from build123d import *

# Parameters (mm, degrees)
BOSS_EXTRU_1_DEPTH = 50
CONG_1_R           = 10


with BuildPart() as part:
    # Esquisse1 → Boss.-Extru.1 (new body)
    with BuildSketch(Plane(origin=(0, 0, 0), x_dir=(1, 0, 0), z_dir=(0, 1, 0))):
        with BuildLine():
            Line((0, 0), (-2, 0))
            ThreePointArc((-2, 0), (6.574510491, 25.388511074), (29, 40.058076335))
            Line((29, 40.058076335), (29, 50.058076335))
            Line((29, 50.058076335), (49, 50.058076335))
            Line((49, 50.058076335), (49, 40.058076335))
            ThreePointArc((49, 40.058076335), (71.425489509, 25.388511074), (80, 0))
            Line((80, 0), (78, 0))
            ThreePointArc((78, 0), (39, 39), (0, 0))
        make_face()
    extrude(amount=BOSS_EXTRU_1_DEPTH)

    # Congé1
    cong_1_edges = [part.edges().sort_by_distance(p)[0] for p in [
        (29, 25, -40.058076335),
        (49, 25, -40.058076335),
    ]]
    fillet(cong_1_edges, radius=CONG_1_R)


solid = part.part
Design review of the part built by this model. Coordinates are the model's own, in mm. A direction names the side the tool comes from. Coordinates: 2 decimals unless noted, no trailing zeros. Order: outer loops, then holes, each group sorted by start corner. A loop starts at its lowest first (then second) coordinate and runs counter-clockwise, first axis right, second up.
Item 1: For line 1 (X direction, y = 21, z = -29); line 2 (X direction, y = 7.5, z = -8); line 3 (X direction, y = 27, z = -47), list the stretches that pass through material, from the lowest coordinate up.
Item 2: Take a section at B-B, the plane y = 44. Write out the cut boundary in (x, z).
Item 3: The part is to be moulded in two halves that separate along X. For faces 3 (the cylindrical face through (39.86, 24.65, -38.99)), 4 (the flat face through (39, 25, -50.058)), 5 (the flat face through (29, 25, -49)), say which applies: pulls with the +X half, pulls with the -X half, needs draft (parallel to the pull), parting line crosses it, or undercut.
Item 4: Take a section at A-A, the plane z = -15. Write out the cut boundary in (x, y).
Item 5: For faces 1 (the cylindrical face through (27.3, 25.35, -41.63)), 2 (the flat face through (49, 25, -49)), list the 3-axis set-ups (+Z, -Z, +X, -X, +Y, -Y) from which the entire face can be reached by the end or side of a thin tool; tool diameter is ignored.
Item 6: For pin 1 Ø3 at (x, y) = (56, 31.5) entering from -Z; pin 2 Ø12 at (x, y) = (40.5, 13.5) entering from +Z; pin 3 Ø3 at (y, z) = (16, -48.5) entering from +X, all flat-tipped, find the tip position at first contact; note any pin that passes through.
Item 7: Take a section at D-D, the plane z = -33. Write out the cut boundary in (x, y).
Item 8: Take a section at C-C, the plane x = 39. Write out the cut boundary in (y, z).
The answers:
1. line 1: x = 9.72 to 12.92, 65.08 to 68.28
1. line 2: x = -1.27 to 0.83, 77.17 to 79.27
1. line 3: x = 29 to 49
2. outline: (-2, 0) arc R41 ccw to (22.92, -38.01) arc R10 cw to (29, -47.21) - (29, -50.06) - (49, -50.06) - (49, -47.21) arc R10 cw to (55.08, -38.01) arc R41 ccw to (80, 0) - (78, 0) arc R39 cw to (0, 0) - close
3. face 3: undercut
3. face 4: needs draft
3. face 5: pulls with the -X half
4. outline: (0.73, 0) - (3, 0) - (3, 50) - (0.73, 50) - close; (75, 0) - (77.27, 0) - (77.27, 50) - (75, 50) - close
5. face 1: -Z, -X, +Y, -Y
5. face 2: -Z, +X, +Y, -Y
6. pin 1: stops at z = -38.28
6. pin 2: stops at z = -38.27
6. pin 3: stops at x = 49
7. outline: (14.27, 0) - (18.22, 0) - (18.22, 50) - (14.27, 50) - close; (59.78, 0) - (63.73, 0) - (63.73, 50) - (59.78, 50) - close
8. outline: (0, -50.06) - (50, -50.06) - (50, -39) - (0, -39) - close
